from build123d import *

# Parameters (mm, degrees)
BOSS_EXTRUDE1_DEPTH = 200
SKETCH2_R           = 19.005135809
SKETCH2_R_2         = 6.150490934
SKETCH2_W           = 14.963877837
SKETCH2_H           = 32.789303583
CUT_EXTRUDE1_DEPTH  = 25


with BuildPart() as part:
    # Sketch1 → Boss-Extrude1 (new body)
    with BuildSketch(Plane(origin=(0, 0, 0), x_dir=(1, 0, 0), z_dir=(0, 1, 0))):
        with BuildLine():
            Line((199.247825531, -25), (-191.027117423, -25))
            ThreePointArc((-191.027117423, -25), (-164.527287911, 7.845509301), (-125.968347388, 25))
            Line((-125.968347388, 25), (134.189055496, 25))
            ThreePointArc((134.189055496, 25), (172.747996019, 7.845509301), (199.247825531, -25))
        make_face()
    extrude(amount=BOSS_EXTRUDE1_DEPTH)

    # Sketch2 → Cut-Extrude1 (cut)
    # profile 1 of 7: a face of its own
    with BuildSketch(Plane(origin=(0, 200, 0), x_dir=(1, 0, 0), z_dir=(0, 1, 0))):
        with Locations(Location((110.270417857, -1.503200416, 0), (0, 0, 270))):
            Circle(SKETCH2_R)
        with Locations(Location((110.270417857, -1.503200416, 0), (0, 0, 270))):
            Circle(SKETCH2_R_2, mode=Mode.SUBTRACT)
    # profile 2 of 7: a face of its own
    with BuildSketch(Plane(origin=(0, 200, 0), x_dir=(1, 0, 0), z_dir=(0, 1, 0))):
        Polygon((-72.460343133, -7.946264371), (-78.025852291, -7.946264371), (-78.025852291, 6.139420836), (-55.550414196, 6.139420836), (-55.550414196, -7.946264371), (-60.107751805, -7.946264371), (-60.107751805, -12.97071102), (-72.460343133, -12.97071102), align=None)
    # profile 3 of 7: a face of its own
    with BuildSketch(Plane(origin=(0, 200, 0), x_dir=(1, 0, 0), z_dir=(0, 1, 0))):
        Polygon((-39.468323041, -7.946264371), (-45.033832199, -7.946264371), (-45.033832199, 6.139420836), (-22.558394104, 6.139420836), (-22.558394104, -7.946264371), (-27.115731714, -7.946264371), (-27.115731714, -12.97071102), (-39.468323041, -12.97071102), align=None)
    # profile 4 of 7: a face of its own
    with BuildSketch(Plane(origin=(0, 200, 0), x_dir=(1, 0, 0), z_dir=(0, 1, 0))):
        Polygon((-4.613365568, -7.946264371), (-10.178874726, -7.946264371), (-10.178874726, 6.139420836), (12.296563369, 6.139420836), (12.296563369, -7.946264371), (7.739225759, -7.946264371), (7.739225759, -12.97071102), (-4.613365568, -12.97071102), align=None)
    # profile 5 of 7: a face of its own
    with BuildSketch(Plane(origin=(0, 200, 0), x_dir=(1, 0, 0), z_dir=(0, 1, 0))):
        Polygon((26.395527633, -7.946264371), (20.830018475, -7.946264371), (20.830018475, 6.139420836), (43.30545657, 6.139420836), (43.30545657, -7.946264371), (38.74811896, -7.946264371), (38.74811896, -12.97071102), (26.395527633, -12.97071102), align=None)
    # profile 6 of 7: a face of its own
    with BuildSketch(Plane(origin=(0, 200, 0), x_dir=(1, 0, 0), z_dir=(0, 1, 0))):
        Polygon((-83.179668167, -12.163715332), (-83.179668167, 4.015448284), (-86.438780262, 4.015448284), (-86.438780262, 8.671322706), (-90.047082939, 8.671322706), (-90.047082939, 12.046831662), (-104.480293646, 12.046831662), (-104.480293646, 8.671322706), (-109.368961789, 8.671322706), (-109.368961789, 4.015448284), (-112.628073884, 4.015448284), (-112.628073884, -12.163715332), align=None)
    # profile 7 of 7: a face of its own
    with BuildSketch(Plane(origin=(0, 200, 0), x_dir=(1, 0, 0), z_dir=(0, 1, 0))):
        with Locations((70.010460819, -4.347820129)):
            Rectangle(SKETCH2_W, SKETCH2_H)
    extrude(amount=-CUT_EXTRUDE1_DEPTH, mode=Mode.SUBTRACT)


solid = part.part
Could you check a few things on this model? Use its own coordinates, in mm. A direction names the side the tool comes from. Round coordinates to 2 decimals unless told otherwise and drop trailing zeros. Write each loop counter-clockwise with the first axis right and the second up, starting at its lowest first coordinate (ties: lowest second). Pieces come first, ordered by that corner, then holes. Notation, with made-up numbers: (-29, 9.25) -> (12, 9.25) arc R14 cw to (12, 23.25) -> close; hole circle Ø11 at (57, 23.25). An arc over 180 degrees is marked (long way). Use a Markdown table: item, result.
1. For pin 1 Ø3.5 at (y, z) = (191, -11) entering from -X; pin 2 Ø2.5 at (y, z) = (189.5, 9) entering from -X; pin 3 Ø1 at (y, z) = (110.5, 12) entering from -X, each with a flat end and sliding along its axis, tell me the tip position at first contact or that it passes through.
Answer key:
| item | result |
|---|---|
| pin 1 | stops at x = -162.65 |
| pin 2 | stops at x = -182.23 |
| pin 3 | stops at x = -183.83 |
2. We'd pull the mould along X, two halves only. Please class faces 3 (the face through (-165, 98.6, -7.48)), 4 (the face through (-98, 175, 0)), 5 (the face through (7, 0, 0)): +X half, -X half, draft (parallel to the pull), parting line (faces both ways), or undercut.
Answer key:
| item | result |
|---|---|
| face 3 | -X half |
| face 4 | undercut |
| face 5 | draft |
3. Which directions (+Z, -Z, +X, -X, +Y, -Y) give clear straight access to the entire face, cutting with the end or side of a thin tool? Please do faces 1 (the face through (7, 200, -11)), 2 (the face through (115, 175, -3)).
Answer key:
| item | result |
|---|---|
| face 1 | +Z, -Z, +X, -X, +Y |
| face 2 | +Y |
4. If we section it at A-A (y = 67): List the corners of the cut face in (x, z) for me.
Answer key:
| item | result |
|---|---|
| outline | (-191.03, 25) arc R90 ccw to (-125.97, -25) -> (134.19, -25) arc R90 ccw to (199.25, 25) -> close |
5. If we section it at B-B (x = 97.5): List the corners of the cut face in (y, z) for me.
Answer key:
| item | result |
|---|---|
| outline | (0, -25) -> (200, -25) -> (200, -12.57) -> (175, -12.57) -> (175, 15.58) -> (200, 15.58) -> (200, 25) -> (0, 25) -> close |
6. Please list where these lines run through material, in increasing order: probe 1 along Y at (x, z) = (96.5, 2); probe 2 along X at (y, z) = (131, 18); probe 3 along Z at (x, y) = (147.5, 97.5).
Answer key:
| item | result |
|---|---|
| probe 1 | y = 0 to 175 |
| probe 2 | x = -187.33 to 195.55 |
| probe 3 | z = -21.48 to 25 |
